The model under review builds one solid part; all positions refer to its coordinate system, in mm. Face numbers are marked on the shaded views. A direction names the side the tool comes from. Round coordinates to 2 decimals unless told otherwise and drop trailing zeros. Loops run counter-clockwise (first coordinate to the right, second up) from the corner with the lowest first, then second, coordinate; pieces in that order, holes last. Notation, with made-up numbers: (-0.5, 25.5) -> (43.5, 25.5) arc R20 cw to (43.5, 32.5) -> close; hole circle Ø2 at (45.25, 74.25). An arc over 180 degrees is marked (long way). Return JSON: item names as keys, results as strings. Group by question number.
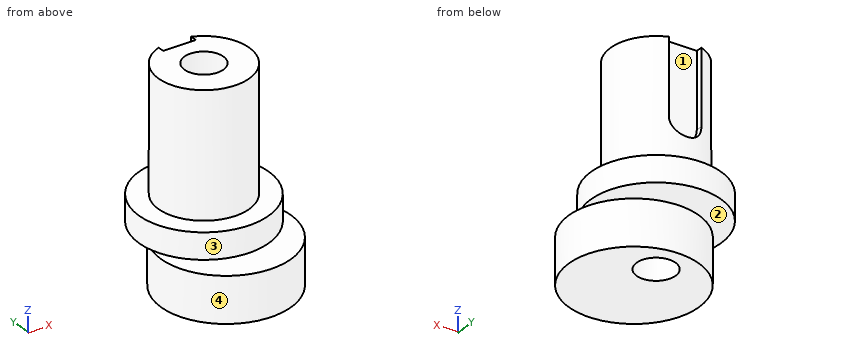
```python
from build123d import *

# Parameters (mm, degrees)
SKETCH1_R           = 10
SKETCH1_R_2         = 3
BOSS_EXTRUDE1_DEPTH = 7
SKETCH2_R           = 10
SKETCH2_R_2         = 3
BOSS_EXTRUDE2_DEPTH = 4
SKETCH3_R           = 7
SKETCH3_R_2         = 3
BOSS_EXTRUDE3_DEPTH = 19
CUT_EXTRUDE1_START  = 20.5
CUT_EXTRUDE1_DEPTH  = 10


with BuildPart() as part:
    # Sketch1 → Boss-Extrude1 (new body)
    with BuildSketch(Plane.XY):
        Circle(SKETCH1_R)
        with Locations((0, 5)):
            Circle(SKETCH1_R_2, mode=Mode.SUBTRACT)
    extrude(amount=BOSS_EXTRUDE1_DEPTH)

    # Sketch2 → Boss-Extrude2 (add)
    with BuildSketch(Plane.XY.offset(7)):
        with Locations((0, 5)):
            Circle(SKETCH2_R)
        with Locations((0, 5)):
            Circle(SKETCH2_R_2, mode=Mode.SUBTRACT)
    extrude(amount=BOSS_EXTRUDE2_DEPTH)

    # Sketch3 → Boss-Extrude3 (add)
    with BuildSketch(Plane.XY.offset(11)):
        with Locations((0, 5)):
            Circle(SKETCH3_R)
        with Locations((0, 5)):
            Circle(SKETCH3_R_2, mode=Mode.SUBTRACT)
    extrude(amount=BOSS_EXTRUDE3_DEPTH)

    # Sketch5 → Cut-Extrude1 (cut)
    with BuildSketch(Plane(origin=(0, 0, 0), x_dir=(1, 0, 0), z_dir=(0, 1, 0)).offset(CUT_EXTRUDE1_START)):
        with BuildLine():
            Line((2.5, -44), (-2.5, -44))
            Line((-2.5, -44), (-2.5, -18.5))
            ThreePointArc((-2.5, -18.5), (0, -16), (2.5, -18.5))
            Line((2.5, -18.5), (2.5, -44))
        make_face()
    extrude(amount=-CUT_EXTRUDE1_DEPTH, mode=Mode.SUBTRACT)


solid = part.part
```
1. We need section C-C, the plane y = 5. Write out the cut boundary in (x, z).
2. We need section D-D, the plane y = 8.5. Write out the cut boundary in (x, z), then the cut area to 3 significant figures.
3. We need section B-B, the plane z = 22.5. Write out the cut boundary in (x, y).
4. For P1, Ø4, axis at x = 7.5, z = 25, coming from the +Y side; P2, Ø3, axis at x = -1.5, z = 25.5, coming from the +Y side; P3, Ø5, axis at x = 0, y = 5, coming from the +Z side; P4, Ø0.5, axis at y = 11.5, z = 24, coming from the +X side, all flat-tipped, find the tip position at first contact; note any pin that passes through.
5. Tool access review of the marked faces 1, 2, 3 and 4: name each direction out of +Z, -Z, +X, -X, +Y, -Y from which nothing blocks a thin tool from reaching the whole face with its end or side.
6. Wall thickness on line 1 (Y direction, x = 0, z = 10.25); line 2 (Y direction, x = 0, z = 6.75); line 3 (X direction, y = 4, z = 4): over which ranges is each line inside the solid? List them lowest first.
7. We need section A-A, the plane x = 0. Write out the cut boundary in (y, z).
Check sheet entries:
{
 "1": {"outline": "(-10, 7) -> (-8.66, 7) -> (-8.66, 0) -> (-3, 0) -> (-3, 30) -> (-7, 30) -> (-7, 11) -> (-10, 11) -> close; (3, 0) -> (8.66, 0) -> (8.66, 7) -> (10, 7) -> (10, 11) -> (7, 11) -> (7, 30) -> (3, 30) -> close"},
 "2": {"outline": "(-9.37, 7) -> (-5.27, 7) -> (-5.27, 0) -> (5.27, 0) -> (5.27, 7) -> (9.37, 7) -> (9.37, 11) -> (6.06, 11) -> (6.06, 30) -> (-6.06, 30) -> (-6.06, 11) -> (-9.37, 11) -> close", "area": "379 mm²"},
 "3": {"outline": "(-2.5, 10.5) -> (-2.5, 11.54) arc R7 ccw (long way) to (2.5, 11.54) -> (2.5, 10.5) -> close; hole circle Ø6 at (0, 5)"},
 "4": {"P1": "stops at y = 9.33", "P2": "stops at y = 11.54", "P3": "passes through", "P4": "stops at x = 3.15"},
 "5": {"face 1": "+Z, +Y", "face 2": "-Z, +Y", "face 3": "+Z", "face 4": "-Z"},
 "6": {"line 1": "y = -5 to 2, 8 to 15", "line 2": "y = -10 to 2, 8 to 10", "line 3": "x = -9.17 to -2.83, 2.83 to 9.17"},
 "7": {"outline": "(-10, 0) -> (2, 0) -> (2, 30) -> (-2, 30) -> (-2, 11) -> (-5, 11) -> (-5, 7) -> (-10, 7) -> close; (8, 0) -> (10, 0) -> (10, 7) -> (15, 7) -> (15, 11) -> (12, 11) -> (12, 16) -> (10.5, 16) -> (10.5, 30) -> (8, 30) -> close"}
}
